```python
from build123d import *

# Parameters (mm, degrees)
PRISM001_DEPTH          = 50
PRISM_DEPTH             = 50
CUBE004_W               = 67
CUBE004_H               = 15
CUBE004_DEPTH           = 15
CUBE004_PLACEMENT_ANGLE = 45
CUBE006_W               = 1
CUBE006_H               = 1.7
CUBE006_DEPTH           = 15
CUBE007_W               = 1
CUBE007_H               = 1.7
CUBE007_DEPTH           = 15
CUBE008_W               = 1
CUBE008_H               = 1.7
CUBE008_DEPTH           = 15
CUBE009_W               = 1
CUBE009_H               = 1.7
CUBE009_DEPTH           = 15
CUBE010_W               = 1
CUBE010_H               = 1.7
CUBE010_DEPTH           = 15
CUBE011_W               = 1
CUBE011_H               = 1.7
CUBE011_DEPTH           = 15
CUBE012_W               = 1
CUBE012_H               = 1.7
CUBE012_DEPTH           = 15
CUBE013_W               = 1
CUBE013_H               = 1.7
CUBE013_DEPTH           = 15
CUBE014_W               = 1
CUBE014_H               = 1.7
CUBE014_DEPTH           = 15
CUBE015_W               = 1
CUBE015_H               = 1.7
CUBE015_DEPTH           = 15
CUBE016_W               = 1
CUBE016_H               = 1.7
CUBE016_DEPTH           = 15
CUBE017_W               = 1
CUBE017_H               = 1.7
CUBE017_DEPTH           = 15
CUBE018_W               = 1
CUBE018_H               = 1.7
CUBE018_DEPTH           = 15
CUBE019_W               = 1
CUBE019_H               = 1.7
CUBE019_DEPTH           = 15
CUBE020_W               = 1
CUBE020_H               = 1.7
CUBE020_DEPTH           = 15
CUBE021_W               = 1
CUBE021_H               = 1.7
CUBE021_DEPTH           = 15
CUBE022_W               = 1
CUBE022_H               = 1.7
CUBE022_DEPTH           = 15
CUBE023_W               = 1
CUBE023_H               = 1.7
CUBE023_DEPTH           = 15
CUBE024_W               = 1
CUBE024_H               = 1.7
CUBE024_DEPTH           = 15
CUBE025_W               = 1
CUBE025_H               = 1.7
CUBE025_DEPTH           = 15
CUBE026_W               = 1
CUBE026_H               = 1.7
CUBE026_DEPTH           = 15
CUBE027_W               = 1
CUBE027_H               = 1.7
CUBE027_DEPTH           = 15
CUBE028_W               = 1
CUBE028_H               = 1.7
CUBE028_DEPTH           = 15
CUBE005_W               = 1
CUBE005_H               = 1.7
CUBE005_DEPTH           = 15
CUBE029_W               = 4
CUBE029_H               = 11
CUBE029_DEPTH           = 15
CUBE030_W               = 13
CUBE030_H               = 13
CUBE030_DEPTH           = 20
CUBE003_W               = 67
CUBE003_H               = 0.55
CUBE003_DEPTH           = 15
CUBE001_W               = 33
CUBE001_H               = 25
CUBE001_DEPTH           = 16
CUBE002_W               = 50
CUBE002_H               = 4
CUBE002_DEPTH           = 16
CUBE_W                  = 33
CUBE_H                  = 15
CUBE_DEPTH              = 16


with BuildPart() as prism001:
    # prism001 → prism001 (new body)
    with BuildSketch(Plane(origin=(-45.5, 0.1, 7.5), x_dir=(1, 0, 0), z_dir=(0, 1, 0))):
        Polygon((1.7, 0), (1.375329, 0.999235), (0.525329, 1.616796), (-0.525329, 1.616796), (-1.375329, 0.999235), (-1.7, 0), (-1.375329, -0.999235), (-0.525329, -1.616796), (0.525329, -1.616796), (1.375329, -0.999235), align=None)
    extrude(amount=PRISM001_DEPTH)


with BuildPart() as group003:
    # prism → prism (new body)
    with BuildSketch(Plane(origin=(-4.5, 0.1, 7.5), x_dir=(1, 0, 0), z_dir=(0, 1, 0))):
        Polygon((1.7, 0), (1.375329, 0.999235), (0.525329, 1.616796), (-0.525329, 1.616796), (-1.375329, 0.999235), (-1.7, 0), (-1.375329, -0.999235), (-0.525329, -1.616796), (0.525329, -1.616796), (1.375329, -0.999235), align=None)
    extrude(amount=PRISM_DEPTH)

    # Group003: union prism001
    add(prism001.part)


with BuildPart() as cube004:
    # cube004 → cube004 (new body)
    with BuildSketch(Plane.XY):
        with Locations((33.5, 7.5)):
            Rectangle(CUBE004_W, CUBE004_H)
    extrude(amount=CUBE004_DEPTH)


with BuildPart() as cube004_1:
    # cube004 placement: moved
    add(cube004.part.moved(Location((-66, 9.5, 12))).rotate(Axis((-66, 9.5, 12), (1, 0, 0)), CUBE004_PLACEMENT_ANGLE))


with BuildPart() as cube006:
    # cube006 → cube006 (new body)
    with BuildSketch(Plane(origin=(-3.1, 8, 3), x_dir=(1, 0, 0), z_dir=(0, 0, 1))):
        with Locations((0.5, 0.85)):
            Rectangle(CUBE006_W, CUBE006_H)
    extrude(amount=CUBE006_DEPTH)


with BuildPart() as cube007:
    # cube007 → cube007 (new body)
    with BuildSketch(Plane(origin=(-5.1, 8, 3), x_dir=(1, 0, 0), z_dir=(0, 0, 1))):
        with Locations((0.5, 0.85)):
            Rectangle(CUBE007_W, CUBE007_H)
    extrude(amount=CUBE007_DEPTH)


with BuildPart() as cube008:
    # cube008 → cube008 (new body)
    with BuildSketch(Plane(origin=(-7.1, 8, 3), x_dir=(1, 0, 0), z_dir=(0, 0, 1))):
        with Locations((0.5, 0.85)):
            Rectangle(CUBE008_W, CUBE008_H)
    extrude(amount=CUBE008_DEPTH)


with BuildPart() as cube009:
    # cube009 → cube009 (new body)
    with BuildSketch(Plane(origin=(-9.1, 8, 3), x_dir=(1, 0, 0), z_dir=(0, 0, 1))):
        with Locations((0.5, 0.85)):
            Rectangle(CUBE009_W, CUBE009_H)
    extrude(amount=CUBE009_DEPTH)


with BuildPart() as cube010:
    # cube010 → cube010 (new body)
    with BuildSketch(Plane(origin=(-11.1, 8, 3), x_dir=(1, 0, 0), z_dir=(0, 0, 1))):
        with Locations((0.5, 0.85)):
            Rectangle(CUBE010_W, CUBE010_H)
    extrude(amount=CUBE010_DEPTH)


with BuildPart() as cube011:
    # cube011 → cube011 (new body)
    with BuildSketch(Plane(origin=(-13.1, 8, 3), x_dir=(1, 0, 0), z_dir=(0, 0, 1))):
        with Locations((0.5, 0.85)):
            Rectangle(CUBE011_W, CUBE011_H)
    extrude(amount=CUBE011_DEPTH)


with BuildPart() as cube012:
    # cube012 → cube012 (new body)
    with BuildSketch(Plane(origin=(-15.1, 8, 3), x_dir=(1, 0, 0), z_dir=(0, 0, 1))):
        with Locations((0.5, 0.85)):
            Rectangle(CUBE012_W, CUBE012_H)
    extrude(amount=CUBE012_DEPTH)


with BuildPart() as cube013:
    # cube013 → cube013 (new body)
    with BuildSketch(Plane(origin=(-17.1, 8, 3), x_dir=(1, 0, 0), z_dir=(0, 0, 1))):
        with Locations((0.5, 0.85)):
            Rectangle(CUBE013_W, CUBE013_H)
    extrude(amount=CUBE013_DEPTH)


with BuildPart() as cube014:
    # cube014 → cube014 (new body)
    with BuildSketch(Plane(origin=(-19.1, 8, 3), x_dir=(1, 0, 0), z_dir=(0, 0, 1))):
        with Locations((0.5, 0.85)):
            Rectangle(CUBE014_W, CUBE014_H)
    extrude(amount=CUBE014_DEPTH)


with BuildPart() as cube015:
    # cube015 → cube015 (new body)
    with BuildSketch(Plane(origin=(-21.1, 8, 3), x_dir=(1, 0, 0), z_dir=(0, 0, 1))):
        with Locations((0.5, 0.85)):
            Rectangle(CUBE015_W, CUBE015_H)
    extrude(amount=CUBE015_DEPTH)


with BuildPart() as cube016:
    # cube016 → cube016 (new body)
    with BuildSketch(Plane(origin=(-23.1, 8, 3), x_dir=(1, 0, 0), z_dir=(0, 0, 1))):
        with Locations((0.5, 0.85)):
            Rectangle(CUBE016_W, CUBE016_H)
    extrude(amount=CUBE016_DEPTH)


with BuildPart() as cube017:
    # cube017 → cube017 (new body)
    with BuildSketch(Plane(origin=(-25.1, 8, 3), x_dir=(1, 0, 0), z_dir=(0, 0, 1))):
        with Locations((0.5, 0.85)):
            Rectangle(CUBE017_W, CUBE017_H)
    extrude(amount=CUBE017_DEPTH)


with BuildPart() as cube018:
    # cube018 → cube018 (new body)
    with BuildSketch(Plane(origin=(-27.1, 8, 3), x_dir=(1, 0, 0), z_dir=(0, 0, 1))):
        with Locations((0.5, 0.85)):
            Rectangle(CUBE018_W, CUBE018_H)
    extrude(amount=CUBE018_DEPTH)


with BuildPart() as cube019:
    # cube019 → cube019 (new body)
    with BuildSketch(Plane(origin=(-29.1, 8, 3), x_dir=(1, 0, 0), z_dir=(0, 0, 1))):
        with Locations((0.5, 0.85)):
            Rectangle(CUBE019_W, CUBE019_H)
    extrude(amount=CUBE019_DEPTH)


with BuildPart() as cube020:
    # cube020 → cube020 (new body)
    with BuildSketch(Plane(origin=(-31.1, 8, 3), x_dir=(1, 0, 0), z_dir=(0, 0, 1))):
        with Locations((0.5, 0.85)):
            Rectangle(CUBE020_W, CUBE020_H)
    extrude(amount=CUBE020_DEPTH)


with BuildPart() as cube021:
    # cube021 → cube021 (new body)
    with BuildSketch(Plane(origin=(-33.1, 8, 3), x_dir=(1, 0, 0), z_dir=(0, 0, 1))):
        with Locations((0.5, 0.85)):
            Rectangle(CUBE021_W, CUBE021_H)
    extrude(amount=CUBE021_DEPTH)


with BuildPart() as cube022:
    # cube022 → cube022 (new body)
    with BuildSketch(Plane(origin=(-35.1, 8, 3), x_dir=(1, 0, 0), z_dir=(0, 0, 1))):
        with Locations((0.5, 0.85)):
            Rectangle(CUBE022_W, CUBE022_H)
    extrude(amount=CUBE022_DEPTH)


with BuildPart() as cube023:
    # cube023 → cube023 (new body)
    with BuildSketch(Plane(origin=(-37.1, 8, 3), x_dir=(1, 0, 0), z_dir=(0, 0, 1))):
        with Locations((0.5, 0.85)):
            Rectangle(CUBE023_W, CUBE023_H)
    extrude(amount=CUBE023_DEPTH)


with BuildPart() as cube024:
    # cube024 → cube024 (new body)
    with BuildSketch(Plane(origin=(-39.1, 8, 3), x_dir=(1, 0, 0), z_dir=(0, 0, 1))):
        with Locations((0.5, 0.85)):
            Rectangle(CUBE024_W, CUBE024_H)
    extrude(amount=CUBE024_DEPTH)


with BuildPart() as cube025:
    # cube025 → cube025 (new body)
    with BuildSketch(Plane(origin=(-41.1, 8, 3), x_dir=(1, 0, 0), z_dir=(0, 0, 1))):
        with Locations((0.5, 0.85)):
            Rectangle(CUBE025_W, CUBE025_H)
    extrude(amount=CUBE025_DEPTH)


with BuildPart() as cube026:
    # cube026 → cube026 (new body)
    with BuildSketch(Plane(origin=(-43.1, 8, 3), x_dir=(1, 0, 0), z_dir=(0, 0, 1))):
        with Locations((0.5, 0.85)):
            Rectangle(CUBE026_W, CUBE026_H)
    extrude(amount=CUBE026_DEPTH)


with BuildPart() as cube027:
    # cube027 → cube027 (new body)
    with BuildSketch(Plane(origin=(-45.1, 8, 3), x_dir=(1, 0, 0), z_dir=(0, 0, 1))):
        with Locations((0.5, 0.85)):
            Rectangle(CUBE027_W, CUBE027_H)
    extrude(amount=CUBE027_DEPTH)


with BuildPart() as cube028:
    # cube028 → cube028 (new body)
    with BuildSketch(Plane(origin=(-47.1, 8, 3), x_dir=(1, 0, 0), z_dir=(0, 0, 1))):
        with Locations((0.5, 0.85)):
            Rectangle(CUBE028_W, CUBE028_H)
    extrude(amount=CUBE028_DEPTH)


with BuildPart() as group001:
    # cube005 → cube005 (new body)
    with BuildSketch(Plane(origin=(-1.1, 8, 3), x_dir=(1, 0, 0), z_dir=(0, 0, 1))):
        with Locations((0.5, 0.85)):
            Rectangle(CUBE005_W, CUBE005_H)
    extrude(amount=CUBE005_DEPTH)

    # Group001: union cube006, cube007, cube008, cube009, cube010, cube011, cube012, cube013, cube014, cube015, cube016, cube017, cube018, cube019, cube020, cube021, cube022, cube023, cube024, cube025, cube026, cube027, cube028
    add(cube006.part)
    add(cube007.part)
    add(cube008.part)
    add(cube009.part)
    add(cube010.part)
    add(cube011.part)
    add(cube012.part)
    add(cube013.part)
    add(cube014.part)
    add(cube015.part)
    add(cube016.part)
    add(cube017.part)
    add(cube018.part)
    add(cube019.part)
    add(cube020.part)
    add(cube021.part)
    add(cube022.part)
    add(cube023.part)
    add(cube024.part)
    add(cube025.part)
    add(cube026.part)
    add(cube027.part)
    add(cube028.part)


with BuildPart() as cube029:
    # cube029 → cube029 (new body)
    with BuildSketch(Plane(origin=(-27, -1, 3), x_dir=(1, 0, 0), z_dir=(0, 0, 1))):
        with Locations((2, 5.5)):
            Rectangle(CUBE029_W, CUBE029_H)
    extrude(amount=CUBE029_DEPTH)


with BuildPart() as cube030:
    # cube030 → cube030 (new body)
    with BuildSketch(Plane(origin=(-31.5, 17, -2), x_dir=(1, 0, 0), z_dir=(0, 0, 1))):
        with Locations((6.5, 6.5)):
            Rectangle(CUBE030_W, CUBE030_H)
    extrude(amount=CUBE030_DEPTH)


with BuildPart() as union:
    # cube003 → cube003 (new body)
    with BuildSketch(Plane(origin=(-66, 9.5, 3), x_dir=(1, 0, 0), z_dir=(0, 0, 1))):
        with Locations((33.5, 0.275)):
            Rectangle(CUBE003_W, CUBE003_H)
    extrude(amount=CUBE003_DEPTH)

    # Group002: union cube004, Group001, cube029, cube030
    add(cube004_1.part)
    add(group001.part)
    add(cube029.part)
    add(cube030.part)

    # union: union Group003
    add(group003.part)


with BuildPart() as cube001:
    # cube001 → cube001 (new body)
    with BuildSketch(Plane(origin=(-41.5, 11, -1), x_dir=(1, 0, 0), z_dir=(0, 0, 1))):
        with Locations((16.5, 12.5)):
            Rectangle(CUBE001_W, CUBE001_H)
    extrude(amount=CUBE001_DEPTH)


with BuildPart() as cube002:
    # cube002 → cube002 (new body)
    with BuildSketch(Plane(origin=(-50, 32, -1), x_dir=(1, 0, 0), z_dir=(0, 0, 1))):
        with Locations((25, 2)):
            Rectangle(CUBE002_W, CUBE002_H)
    extrude(amount=CUBE002_DEPTH)


with BuildPart() as difference:
    # cube → cube (new body)
    with BuildSketch(Plane(origin=(-41.5, 0, -1), x_dir=(1, 0, 0), z_dir=(0, 0, 1))):
        with Locations((16.5, 7.5)):
            Rectangle(CUBE_W, CUBE_H)
    extrude(amount=CUBE_DEPTH)

    # Group: union cube001, cube002
    add(cube001.part)
    add(cube002.part)

    # difference: cut union
    add(union.part, mode=Mode.SUBTRACT)


solid = difference.part
```
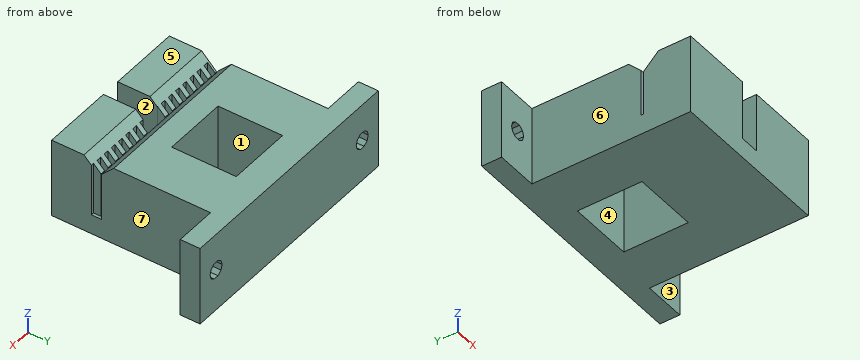
Geometry check sheet. Reference: the model listing, model coordinates, mm. Face numbers are marked on the shaded views. A direction names the side the tool comes from. Give positions to 0.01 mm unless a question says otherwise; leave off trailing zeros. Write each loop counter-clockwise with the first axis right and the second up, starting at its lowest first coordinate (ties: lowest second). Pieces come first, ordered by that corner, then holes. Notation, with made-up numbers: (-36.5, 36.25) -> (-5.5, 36.25) arc R22 ccw to (-5.5, 57.25) -> close; hole circle Ø1 at (4, 60.5). An arc over 180 degrees is marked (long way). Use one line per item in the form item = value.
Item 1: Sectioned sample at B-B on y = 24.5. Enter the section's corners in (x, z), plus the area to 3 significant figures.
Results list:
outline = (-41.5, -1) -> (-31.5, -1) -> (-31.5, 15) -> (-41.5, 15) -> close; (-18.5, -1) -> (-8.5, -1) -> (-8.5, 15) -> (-18.5, 15) -> close
area = 320 mm2
Item 2: Sectioned sample at D-D on y = 34.5. Enter the section's corners in (x, z).
Results list:
outline = (-50, -1) -> (0, -1) -> (0, 15) -> (-50, 15) -> close; hole (-47.2, 7.5) -> (-46.88, 6.5) -> (-46.03, 5.88) -> (-44.97, 5.88) -> (-44.12, 6.5) -> (-43.8, 7.5) -> (-44.12, 8.5) -> (-44.97, 9.12) -> (-46.03, 9.12) -> (-46.88, 8.5) -> close; hole (-6.2, 7.5) -> (-5.88, 6.5) -> (-5.03, 5.88) -> (-3.97, 5.88) -> (-3.12, 6.5) -> (-2.8, 7.5) -> (-3.12, 8.5) -> (-3.97, 9.12) -> (-5.03, 9.12) -> (-5.88, 8.5) -> close
Item 3: Depth check by flat-ended pin: pin 1 Ø5 at (x, z) = (-20, 8.5) entering from -Y; pin 2 Ø1.2 at (y, z) = (9, 7) entering from +X; pin 3 Ø0.8 at (y, z) = (8.5, 8) entering from -X; pin 4 Ø2.5 at (y, z) = (5.5, 8.5) entering from +X. Enter the tip coordinate at first touch or a pass-through.
Results list:
pin_1 = 0
pin_2 = -9.1
pin_3 = -41.5
pin_4 = -8.5
Item 4: Mould release check, pull along X, two halves, no side actions. Record for the marked faces 4, 5, 6 and 7: released by +X, released by -X, zero draft, split by the parting line, or undercut.
Results list:
face_4 = undercut
face_5 = zero draft
face_6 = released by -X
face_7 = released by +X
Item 5: Sectioned sample at A-A on z = 2.25. Enter the section's corners in (x, y), plus the area to 3 significant figures.
Results list:
outline = (-50, 32) -> (-41.5, 32) -> (-41.5, 0) -> (-8.5, 0) -> (-8.5, 32) -> (0, 32) -> (0, 36) -> (-50, 36) -> close; hole (-31.5, 17) -> (-18.5, 17) -> (-18.5, 30) -> (-31.5, 30) -> close
area = 1,090 mm2
Item 6: Scan lines: line 1 (Y direction, x = -19.5, z = 4.25); line 2 (X direction, y = 22, z = 3.5); line 3 (Y direction, x = -38, z = 9). Record each from-to range of solid material in increasing order.
Results list:
line_1 = 0 to 9.5, 10.05 to 17, 30 to 36
line_2 = -41.5 to -31.5, -18.5 to -8.5
line_3 = 0 to 9.5, 10.05 to 36
Item 7: Access from +Z, -Z, +X, -X, +Y, -Y to the whole of each face (thin tool, end or side, straight path). Record for the marked faces 1, 2 and 3.
Results list:
face_1 = +Z, -Z
face_2 = +Z, -Y
face_3 = +Z, -Z, +X, -Y
Item 8: Sectioned sample at C-C on x = -26. Enter the section's corners in (y, z).
Results list:
outline = (0, -1) -> (17, -1) -> (17, 15) -> (12.5, 15) -> (10.05, 12.55) -> (10.05, 3) -> (0, 3) -> close; (30, -1) -> (36, -1) -> (36, 15) -> (30, 15) -> close
